The model under review builds one solid part; all positions refer to its coordinate system, in mm. Face numbers are marked on the shaded views. A direction names the side the tool comes from. Give positions to 0.01 mm unless a question says otherwise; leave off trailing zeros. Order: outer loops, then holes, each group sorted by start corner. A loop starts at its lowest first (then second) coordinate and runs counter-clockwise, first axis right, second up. Notation, with made-up numbers: (3, 32.25) - (26, 32.25) arc R25 ccw to (26, 53.25) - close; hole circle Ø7 at (-29, 5.5). An arc over 180 degrees is marked (long way). Use a Markdown table: item, result. Add a question column.
```python
from build123d import *

# Parameters (mm, degrees)
SKETCH1_W           = 40
SKETCH1_H           = 40
BOSS_EXTRUDE1_DEPTH = 40
CUT_EXTRUDE1_DEPTH  = 71
SKETCH3_W           = 20
SKETCH3_H           = 20
CUT_EXTRUDE2_DEPTH  = 71
BOSS_EXTRUDE2_DEPTH = 20


with BuildPart() as part:
    # Sketch1 → Boss-Extrude1 (new body)
    with BuildSketch(Plane.XY):
        with Locations((20, 20)):
            Rectangle(SKETCH1_W, SKETCH1_H)
    extrude(amount=BOSS_EXTRUDE1_DEPTH)

    # Sketch2 → Cut-Extrude1 (cut)
    with BuildSketch(Plane.ZY):
        with BuildLine():
            Line((20, 40), (0, 40))
            Line((0, 40), (0, 20))
            ThreePointArc((0, 20), (5.857864376, 34.142135624), (20, 40))
        make_face()
        with BuildLine():
            Line((40, 40), (20, 40))
            ThreePointArc((20, 40), (34.142135624, 34.142135624), (40, 20))
            Line((40, 20), (40, 40))
        make_face()
        with BuildLine():
            Line((40, 0), (40, 20))
            ThreePointArc((40, 20), (34.142135624, 5.857864376), (20, 0))
            Line((20, 0), (40, 0))
        make_face()
        with BuildLine():
            ThreePointArc((20, 0), (5.857864376, 5.857864376), (0, 20))
            Line((0, 20), (0, 0))
            Line((0, 0), (20, 0))
        make_face()
    extrude(amount=-CUT_EXTRUDE1_DEPTH, mode=Mode.SUBTRACT)

    # Sketch3 → Cut-Extrude2 (cut)
    with BuildSketch(Plane.XY):
        with Locations((20, 30)):
            Rectangle(SKETCH3_W, SKETCH3_H)
    extrude(amount=CUT_EXTRUDE2_DEPTH, mode=Mode.SUBTRACT)

    # Sketch4 → Boss-Extrude2 (add)
    with BuildSketch(Plane(origin=(10, 0, 0), x_dir=(0, 0, -1), z_dir=(1, 0, 0))):
        Polygon((-40, 20), (-20, 20), (-20, 40), align=None)
        Polygon((-20, 40), (-20, 20), (0, 20), align=None)
    extrude(amount=BOSS_EXTRUDE2_DEPTH)


solid = part.part
```
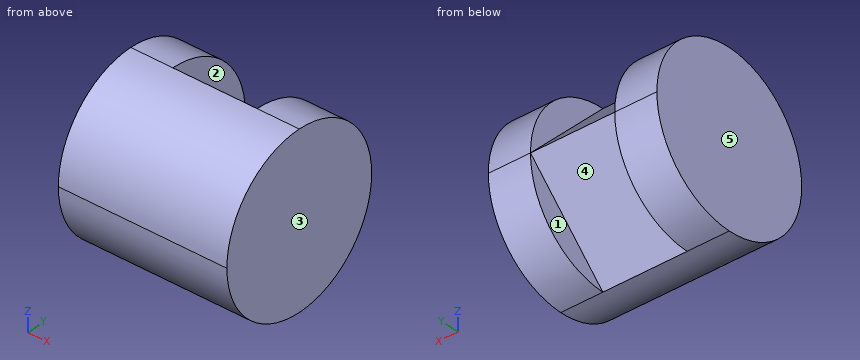
Q1. Wall thickness on probe 1 along X at (y, z) = (29, 34.5); probe 2 along Y at (x, z) = (5, 19.5); probe 3 along Z at (x, y) = (16, 13.5): over which ranges is each line inside the solid? List them lowest first.
Q2. We need section A-A (y = 36). Write out the cut boundary in (x, z), plus the area to 3 significant figures.
Q3. We need section D-D (z = 18). Write out the cut boundary in (x, y), plus the area to 3 significant figures.
Q4. We need section B-B (z = 23). Write out the cut boundary in (x, y), plus the area to 3 significant figures.
Q5. Draft analysis for pull direction X (two halves, no side actions). For the marked faces 3, 4 and 5, state which applies: pulls with the +X half, pulls with the -X half, needs draft (parallel to the pull), parting line crosses it, or undercut.
Q6. We need section C-C (x = 17). Write out the cut boundary in (y, z).
Q7. Clearance check with flat-ended pins moving along their axes: P1, Ø5, axis at x = 6.5, z = 13.5, coming from the +Y side; P2, Ø1, axis at x = 18, y = 16, coming from the +Z side; P3, Ø2, axis at x = 26, z = 31, coming from the +Y side. State where each tip first meets the part, or that it passes through.
Q8. Machinability: for the marked faces 1 and 2, which of the approach directions +Z, -Z, +X, -X, +Y, -Y give a long, thin tool a straight path to every point of the face, cutting with its end or side? Answer none if there is none.
Here are the results:
| question | item | result |
|---|---|---|
| 1 | probe 1 | 0 to 10, 30 to 40 |
| 1 | probe 2 | 0.01 to 39.99 |
| 1 | probe 3 | 1.09 to 38.91 |
| 2 | outline | (0, 8) - (10, 8) - (10, 16) - (30, 16) - (30, 8) - (40, 8) - (40, 32) - (30, 32) - (30, 24) - (10, 24) - (10, 32) - (0, 32) - close |
| 2 | area | 640 mm2 |
| 3 | outline | (0, 0.1) - (40, 0.1) - (40, 39.9) - (30, 39.9) - (30, 38) - (10, 38) - (10, 39.9) - (0, 39.9) - close |
| 3 | area | 1,550 mm2 |
| 4 | outline | (0, 0.23) - (40, 0.23) - (40, 39.77) - (30, 39.77) - (30, 37) - (10, 37) - (10, 39.77) - (0, 39.77) - close |
| 4 | area | 1,530 mm2 |
| 5 | face 3 | pulls with the +X half |
| 5 | face 4 | undercut |
| 5 | face 5 | pulls with the -X half |
| 6 | outline | (20, 0) - (40, 20) - (20, 40) arc R20 ccw to start |
| 7 | P1 | y = 39.6 |
| 7 | P2 | z = 39.69 |
| 7 | P3 | y = 30 |
| 8 | face 1 | -Z, +Y |
| 8 | face 2 | +Z, +Y |
